Source: CAD feature listing. Evaluate the final solid. Frame: model axes, mm. Face numbers are marked on the shaded views. A direction names the side the tool comes from. Give positions to 0.01 mm unless a question says otherwise; leave off trailing zeros. Order: outer loops, then holes, each group sorted by start corner. A loop starts at its lowest first (then second) coordinate and runs counter-clockwise, first axis right, second up.
1) Draft query along Z for the marked faces 1, 2 and 3. Return one class per face: released by +Z, released by -Z, zero draft, split by the parting line, or undercut.
2) Access query for the marked faces 4 and 5. Directions: +Z, -Z, +X, -X, +Y, -Y. A direction counts if a zero-diameter tool reaches every point of the face in a straight line with its end or side. Return the directions, or none.
3) Section B-B, the plane y = 8.25. Return loops of the section in (x, z).
4) Material intervals for line 1 (X direction, y = 2.75, z = -62); line 2 (Z direction, x = 105, y = 5.5); line 3 (Z direction, x = 138, y = 3.75), sorted ascending.
5) Section A-A, the plane x = 95. Return loops of the section in (y, z), plus the area to 3 significant figures.
6) First-contact query: P1, Ø5, axis at y = 7.5, z = -18.5, coming from the +X side; P2, Ø0.9, axis at y = 1.5, z = -42, coming from the +X side; P3, Ø8, axis at x = 111.5, z = -66.5, coming from the +Y side. Flat tips, straight axial feed; report the tip coordinate or a pass-through.
7) Section C-C, the plane z = -29.5. Return loops of the section in (x, y).
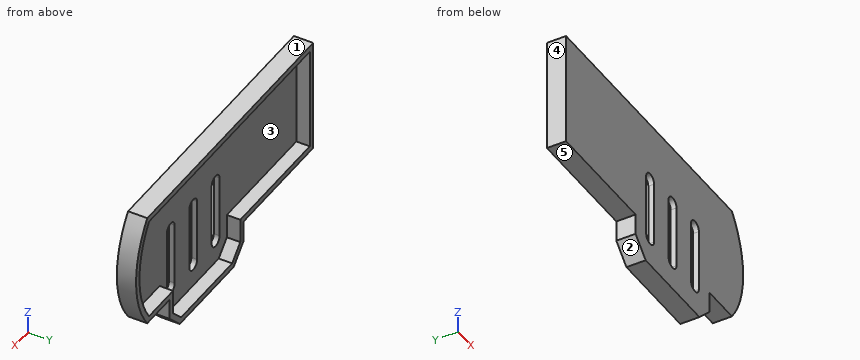
```python
from build123d import *

# Parameters (mm, degrees)
EXTRUDE_1_DEPTH     = 10
CUT_EXTRUDE_1_DEPTH = 7


with BuildPart() as part:
    # Эскиз1 → Бобышка-Вытянуть1 (new body)
    with BuildSketch(Plane(origin=(0, 0, 0), x_dir=(1, 0, 0), z_dir=(0, 1, 0))):
        with BuildLine():
            Line((0, 0), (0, 60))
            Line((0, 60), (62, 60))
            Line((62, 60), (62, 71))
            Line((62, 71), (71, 80))
            Line((71, 80), (119, 80))
            Line((119, 80), (128, 71))
            Line((128, 71), (128, 60))
            Line((128, 60), (148, 60))
            ThreePointArc((148, 60), (158, 30), (148, 0))
            Line((148, 0), (0, 0))
        make_face()
        with BuildLine():
            Line((98.5, 64.5), (98.5, 31.5))
            ThreePointArc((98.5, 31.5), (95, 28), (91.5, 31.5))
            Line((91.5, 31.5), (91.5, 64.5))
            ThreePointArc((91.5, 64.5), (95, 68), (98.5, 64.5))
        make_face(mode=Mode.SUBTRACT)
        with BuildLine():
            Line((78.5, 64.5), (78.5, 31.5))
            ThreePointArc((78.5, 31.5), (75, 28), (71.5, 31.5))
            Line((71.5, 31.5), (71.5, 64.5))
            ThreePointArc((71.5, 64.5), (75, 68), (78.5, 64.5))
        make_face(mode=Mode.SUBTRACT)
        with BuildLine():
            Line((111.5, 64.5), (111.5, 31.5))
            ThreePointArc((111.5, 31.5), (115, 28), (118.5, 31.5))
            Line((118.5, 31.5), (118.5, 64.5))
            ThreePointArc((118.5, 64.5), (115, 68), (111.5, 64.5))
        make_face(mode=Mode.SUBTRACT)
    extrude(amount=EXTRUDE_1_DEPTH)

    # Эскиз3 → Вырез-Вытянуть1 (cut)
    with BuildSketch(Plane(origin=(0, 10, 0), x_dir=(1, 0, 0), z_dir=(0, 1, 0))):
        with BuildLine():
            Line((125, 57), (125, 69.757359313))
            Line((125, 69.757359313), (117.757359313, 77))
            Line((117.757359313, 77), (72.242640687, 77))
            Line((72.242640687, 77), (65, 69.757359313))
            Line((65, 69.757359313), (65, 57))
            Line((65, 57), (3, 57))
            Line((3, 57), (3, 3))
            Line((3, 3), (146.470768123, 3))
            ThreePointArc((146.470768123, 3), (155, 30), (146.470768123, 57))
            Line((146.470768123, 57), (125, 57))
        make_face()
    extrude(amount=-CUT_EXTRUDE_1_DEPTH, mode=Mode.SUBTRACT)


solid = part.part
```
From the geometry:
1. face 1: released by +Z
1. face 2: released by -Z
1. face 3: undercut
2. face 4: +Z, -Z, -X, +Y, -Y
2. face 5: -Z, -X, +Y, -Y
3. outline: (0, -60) - (62, -60) - (62, -71) - (71, -80) - (119, -80) - (128, -71) - (128, -60) - (148, -60) arc R50 ccw to (148, 0) - (0, 0) - close; hole (3, -57) - (65, -57) - (65, -69.76) - (72.24, -77) - (117.76, -77) - (125, -69.76) - (125, -57) - (146.47, -57) arc R47 ccw to (146.47, -3) - (3, -3) - close
4. line 1: x = 62 to 71.5, 78.5 to 91.5, 98.5 to 111.5, 118.5 to 128
4. line 2: z = -80 to -77, -3 to 0
4. line 3: z = -60 to -57, -3 to 0
5. outline: (0, -80) - (10, -80) - (10, -77) - (3, -77) - (3, -68) - (0, -68) - close; (0, -28) - (3, -28) - (3, -3) - (10, -3) - (10, 0) - (0, 0) - close
5. area: 162 mm2
6. P1: stops at x = 157.18
6. P2: stops at x = 156.65
6. P3: stops at y = 3
7. outline: (0, 0) - (72.13, 0) - (72.13, 3) - (3, 3) - (3, 10) - (0, 10) - close; (77.87, 0) - (92.13, 0) - (92.13, 3) - (77.87, 3) - close; (97.87, 0) - (112.13, 0) - (112.13, 3) - (97.87, 3) - close; (117.87, 0) - (158, 0) - (158, 10) - (155, 10) - (155, 3) - (117.87, 3) - close
